from build123d import *

# Parameters (mm, degrees)
SKETCH1_W           = 260
SKETCH1_H           = 75
BOSS_EXTRUDE1_DEPTH = 6
CHAMFER1_SIZE       = 5
FILLET1_R           = 5
SKETCH2_W           = 260
SKETCH2_H           = 67
BOSS_EXTRUDE2_DEPTH = 40
CUT_EXTRUDE1_DEPTH  = 261
SKETCH4_W           = 10
SKETCH4_H           = 67
CUT_EXTRUDE3_DEPTH  = 5.5
CUT_EXTRUDE4_DEPTH  = 35
SKETCH6_R           = 2.5
CUT_EXTRUDE5_DEPTH  = 6.5
SKETCH7_R           = 3
CUT_EXTRUDE6_DEPTH  = 5


with BuildPart() as part:
    # Sketch1 → Boss-Extrude1 (new body)
    with BuildSketch(Plane(origin=(0, 0, 0), x_dir=(1, 0, 0), z_dir=(0, 1, 0))):
        with Locations((130, 37.5)):
            Rectangle(SKETCH1_W, SKETCH1_H)
    extrude(amount=BOSS_EXTRUDE1_DEPTH)

    # Chamfer1
    chamfer1_edges = [part.edges().sort_by_distance(p)[0] for p in [
        (260, 3, -75),
        (260, 3, 0),
    ]]
    chamfer(chamfer1_edges, length=CHAMFER1_SIZE)

    # Fillet1
    fillet1_edges = [part.edges().sort_by_distance(p)[0] for p in [
        (0, 3, -75),
        (0, 3, 0),
    ]]
    fillet(fillet1_edges, radius=FILLET1_R)

    # Sketch2 → Boss-Extrude2 (add)
    with BuildSketch(Plane(origin=(0, 6, 0), x_dir=(1, 0, 0), z_dir=(0, 1, 0))):
        with Locations((130, 37.5)):
            Rectangle(SKETCH2_W, SKETCH2_H)
    extrude(amount=BOSS_EXTRUDE2_DEPTH)

    # Sketch3 → Cut-Extrude1 (cut, through all)
    with BuildSketch(Plane.ZY):
        Polygon((-66, 46), (-66, 44.5), (-68.5, 44.5), (-68.5, 40.5), (-6.5, 40.5), (-6.5, 44.5), (-9, 44.5), (-9, 46), align=None)
    extrude(amount=-CUT_EXTRUDE1_DEPTH, mode=Mode.SUBTRACT)

    # Sketch4 → Cut-Extrude3 (cut)
    with BuildSketch(Plane(origin=(0, 46, 0), x_dir=(1, 0, 0), z_dir=(0, 1, 0))):
        with Locations((5, 37.5)):
            Rectangle(SKETCH4_W, SKETCH4_H)
    extrude(amount=-CUT_EXTRUDE3_DEPTH, mode=Mode.SUBTRACT)

    # Sketch5 → Cut-Extrude4 (cut)
    with BuildSketch(Plane(origin=(0, 40.5, 0), x_dir=(1, 0, 0), z_dir=(0, 1, 0))):
        Polygon((14, 63.5), (14, 53.5), (118.5, 53.5), (118.5, 56), (210.5, 56), (210.5, 61), (118.5, 61), (118.5, 63.5), align=None)
        Polygon((54, 21.5), (54, 11.5), (158.5, 11.5), (158.5, 14), (250.5, 14), (250.5, 19), (158.5, 19), (158.5, 21.5), align=None)
    extrude(amount=-CUT_EXTRUDE4_DEPTH, mode=Mode.SUBTRACT)

    # Sketch6 → Cut-Extrude5 (cut, through all)
    with BuildSketch(Plane(origin=(0, 5.5, 0), x_dir=(1, 0, 0), z_dir=(0, 1, 0))):
        with Locations((208, 58.5)):
            Circle(SKETCH6_R)
        with Locations((248, 16.5)):
            Circle(SKETCH6_R)
    extrude(amount=-CUT_EXTRUDE5_DEPTH, mode=Mode.SUBTRACT)

    # Sketch7 → Cut-Extrude6 (cut)
    with BuildSketch(Plane.XZ):
        with Locations((170, -37.5)):
            Circle(SKETCH7_R)
    extrude(amount=-CUT_EXTRUDE6_DEPTH, mode=Mode.SUBTRACT)


solid = part.part
Model file for the job. Use its own axes, mm. A direction names the side the tool comes from. Coordinates: 2 decimals unless noted, no trailing zeros. Write each loop counter-clockwise with the first axis right and the second up, starting at its lowest first coordinate (ties: lowest second). Pieces come first, ordered by that corner, then holes. Notation, with made-up numbers: (64.25, 49.25) -> (118.25, 49.25) arc R9 cw to (118.25, 59.25) -> close; hole circle Ø6 at (4, 13). An arc over 180 degrees is marked (long way). One line per item, written item: value. Start each with the question number.
1) Flat gauge pins, fed straight in: pin 1 Ø6 at (x, y) = (226.5, 29) entering from -Z; pin 2 Ø2 at (x, z) = (249, -17.5) entering from +Y (3 decimals); pin 3 Ø6 at (x, y) = (30, 16.5) entering from +Z; pin 4 Ø10 at (x, z) = (207.5, -49) entering from +Y. Where does each tip first touch, or does it go through?
2) Probe probe 1 along Z at (x, y) = (86, 31); probe 2 along Z at (x, y) = (121, 7.5); probe 3 along Z at (x, y) = (190, 42.5). List the from-to ranges inside material, lowest first.
3) Slice it at B-B on x = 70. Write the cut outline in (y, z).
4) Which spindle directions (+Z, -Z, +X, -X, +Y, -Y) get a long thin tool onto all of the face, cutting with end or side? Do faces 1 (the face through (210.385, 2.788, -59.251)), 2 (the face through (204, 23, -14)), 3 (the face through (172.86, 2.46, -36.6)), 4 (the face through (10, 44, -6)). Say none if no direction does.
5) Slice it at C-C on z = -37.5. Write the cut outline in (x, y), then the cut area to 3 significant figures.
6) Slice it at D-D on x = 170. Write the cut outline in (y, z).
7) Slice it at A-A on y = 8.5. Write the cut outline in (x, z).
8) Pull direction X, two halves, no side cores. Call faces 5 (the face through (0, 20, -37)), 6 (the face through (260, 23, -37)), 7 (the face through (128, 26, -71)), 8 (the face through (165, 23, -61)): +X half, -X half, draft (parallel to the pull), parting line (faces both ways), or undercut.
Answers follow:
1. pin 1: z = -71
1. pin 2: through
1. pin 3: z = -4
1. pin 4: y = 40.5
2. probe 1: -71 to -63.5, -53.5 to -21.5, -11.5 to -4
2. probe 2: -71 to -61, -56 to -21.5, -11.5 to -4
2. probe 3: -71 to -68.5, -6.5 to -4
3. outline: (0, -75) -> (6, -75) -> (6, -71) -> (46, -71) -> (46, -66) -> (44.5, -66) -> (44.5, -68.5) -> (40.5, -68.5) -> (40.5, -63.5) -> (5.5, -63.5) -> (5.5, -53.5) -> (40.5, -53.5) -> (40.5, -21.5) -> (5.5, -21.5) -> (5.5, -11.5) -> (40.5, -11.5) -> (40.5, -6.5) -> (44.5, -6.5) -> (44.5, -9) -> (46, -9) -> (46, -4) -> (6, -4) -> (6, 0) -> (0, 0) -> close
4. face 1: +Y, -Y
4. face 2: +Y
4. face 3: -Y
4. face 4: +Z, -Z, -X, +Y
5. outline: (0, 0) -> (167, 0) -> (167, 5) -> (173, 5) -> (173, 0) -> (260, 0) -> (260, 40.5) -> (0, 40.5) -> close
5. area: 10,500 mm2
6. outline: (0, -75) -> (6, -75) -> (6, -71) -> (46, -71) -> (46, -66) -> (44.5, -66) -> (44.5, -68.5) -> (40.5, -68.5) -> (40.5, -61) -> (5.5, -61) -> (5.5, -56) -> (40.5, -56) -> (40.5, -19) -> (5.5, -19) -> (5.5, -14) -> (40.5, -14) -> (40.5, -6.5) -> (44.5, -6.5) -> (44.5, -9) -> (46, -9) -> (46, -4) -> (6, -4) -> (6, 0) -> (0, 0) -> (0, -34.5) -> (5, -34.5) -> (5, -40.5) -> (0, -40.5) -> close
7. outline: (0, -71) -> (260, -71) -> (260, -4) -> (0, -4) -> close; hole (14, -63.5) -> (118.5, -63.5) -> (118.5, -61) -> (210.5, -61) -> (210.5, -56) -> (118.5, -56) -> (118.5, -53.5) -> (14, -53.5) -> close; hole (54, -21.5) -> (158.5, -21.5) -> (158.5, -19) -> (250.5, -19) -> (250.5, -14) -> (158.5, -14) -> (158.5, -11.5) -> (54, -11.5) -> close
8. face 5: -X half
8. face 6: +X half
8. face 7: draft
8. face 8: undercut
